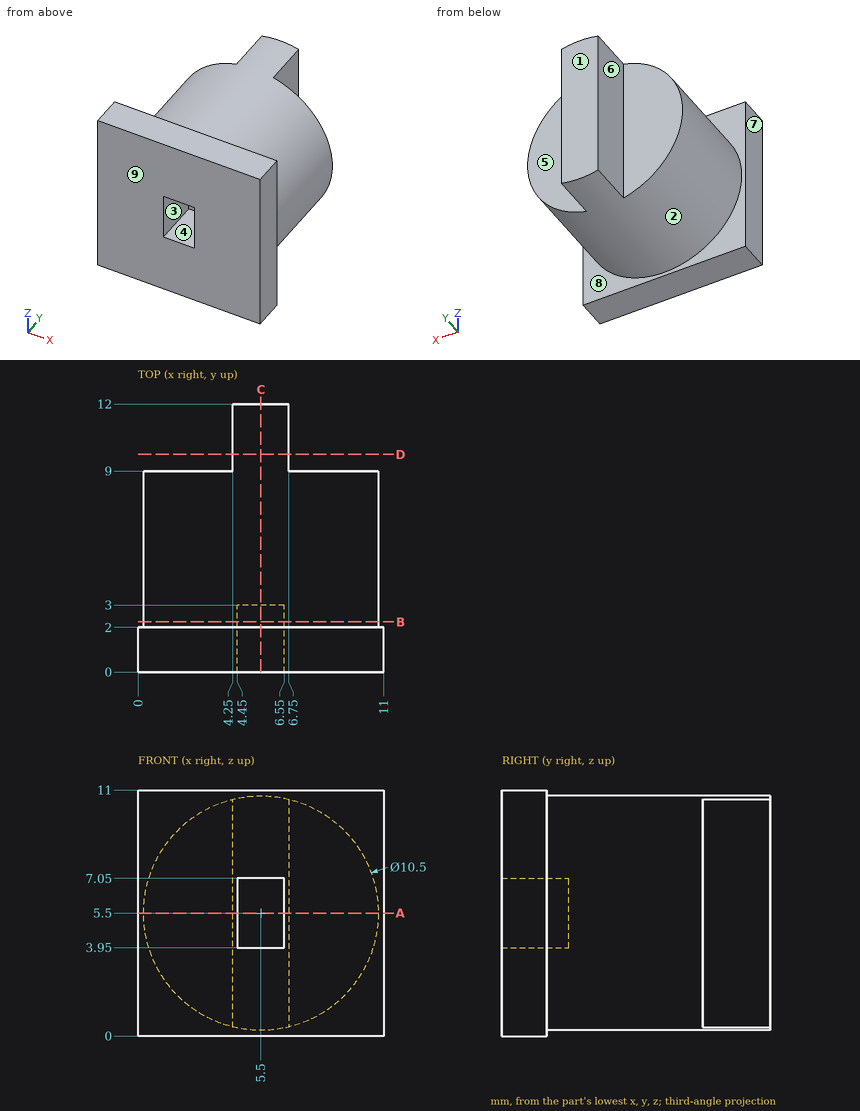
Check sheet for the drawn part. Datum: minimum x, y, z corner. Units: mm. A direction names the side the tool comes from. Round coordinates to 2 decimals unless told otherwise and drop trailing zeros. Order: outer loops, then holes, each group sorted by start corner. A loop starts at its lowest first (then second) coordinate and runs counter-clockwise, first axis right, second up.
1) Section check B-B (y = 2.25). Record the boundary of the cut face in (x, z).
2) Section check A-A (z = 5.5). Record the boundary of the cut face in (x, y).
3) Section check C-C (x = 5.5). Record the boundary of the cut face in (y, z), and give its area (3 significant figures).
4) Tool access check on the marked faces 5, 6, 7, 8 and 9. Record the directions out of +Z, -Z, +X, -X, +Y, -Y that give a thin tool (end or side, any length) a straight path to the whole face; none if there is none.
5) Go/stop test with flat-tipped pins: pin 1 Ø1 at (x, y) = (3.5, 5.5) entering from +Z; pin 2 Ø1.5 at (y, z) = (11, 7.5) entering from +X; pin 3 Ø3.5 at (y, z) = (11, 6) entering from -X. Record where each tip stops, or that it passes through.
6) Section check D-D (y = 9.75). Record the boundary of the cut face in (x, z), and give its area (3 significant figures).
7) Mould release check, pull along X, two halves, no side actions. Record for the marked faces 1, 2, 3 and 4: +X half, -X half, draft (parallel to the pull), parting line (faces both ways), or undercut.
8) Scan lines: line 1 (Y direction, x = 9.75, z = 5); line 2 (Y direction, x = 1.25, z = 0.75); line 3 (Z direction, x = 5.5, y = 11). Record each from-to range of solid material in increasing order.
Result:
1. outline: circle Ø10.5 at (5.5, 5.5); hole (4.45, 3.95) - (6.55, 3.95) - (6.55, 7.05) - (4.45, 7.05) - close
2. outline: (0, 0) - (4.45, 0) - (4.45, 3) - (6.55, 3) - (6.55, 0) - (11, 0) - (11, 2) - (10.75, 2) - (10.75, 9) - (6.75, 9) - (6.75, 12) - (4.25, 12) - (4.25, 9) - (0.25, 9) - (0.25, 2) - (0, 2) - close
3. outline: (0, 0) - (2, 0) - (2, 0.25) - (12, 0.25) - (12, 10.75) - (2, 10.75) - (2, 11) - (0, 11) - (0, 7.05) - (3, 7.05) - (3, 3.95) - (0, 3.95) - close
3. area: 118 mm2
4. face 5: +Z, -Z, +X, +Y
4. face 6: +Z, -Z, -X, +Y
4. face 7: +Z, -Z, -X, +Y, -Y
4. face 8: +Y
4. face 9: +Z, -Z, +X, -X, -Y
5. pin 1: stops at z = 10.53
5. pin 2: stops at x = 6.75
5. pin 3: stops at x = 4.25
6. outline: (4.25, 0.4) arc R5.25 ccw to (6.75, 0.4) - (6.75, 10.6) arc R5.25 ccw to (4.25, 10.6) - close
6. area: 26.0 mm2
7. face 1: draft
7. face 2: parting line
7. face 3: undercut
7. face 4: undercut
8. line 1: y = 0 to 9
8. line 2: y = 0 to 2
8. line 3: z = 0.25 to 10.75
